Could you check a few things on this model? Use its own coordinates, in mm. A direction names the side the tool comes from. Give positions to 0.01 mm unless a question says otherwise; leave off trailing zeros. Order: outer loops, then holes, each group sorted by start corner. A loop starts at its lowest first (then second) coordinate and runs counter-clockwise, first axis right, second up.
(1) Imagine slicing it at A-A, the plane z = 10. Write out the boundary of the cut face in (x, y).
(2) Imagine slicing it at C-C, the plane z = 67.5. Write out the boundary of the cut face in (x, y).
(3) Imagine slicing it at D-D, the plane y = 195. Write out the boundary of the cut face in (x, z), then the cut area to 3 significant figures.
(4) If we mould it in two halves opening along Z, with no side actions, what happens to faces 1 (the cylindrical face through (-175.427, 194.12, 88.496)), 2 (the cylindrical face through (-215.896, 224.268, 60.035)), 3 (the flat face through (-177.399, 209, 45))? For each: released by +Z, released by -Z, zero draft, split by the parting line, or undercut.
(5) If I drill on probe 1 along Z at (x, y) = (-183, 211); probe 2 along Y at (x, z) = (-174.7, 80); probe 3 along X at (y, z) = (222.5, 67), over which ranges is the centre line in solid material (lowest first)?
(6) Will these pins go through, and if not, where does the flat tip stop? pin 1 (4 mm diameter, centred on x = -190.45, y = 215.17, fed in from +Z); pin 2 (1.4 mm diameter, centred on x = -202.62, y = 206.36, fed in from +Z); pin 3 (3 mm diameter, centred on x = -196.676, y = 214.585, fed in from -Z).
(7) Imagine slicing it at B-B, the plane y = 204. Write out the boundary of the cut face in (x, z), then the cut area to 3 significant figures.
(8) On a 3-axis mill with a long thin cutter (end or side, diameter ignored), from which of +Z, -Z, +X, -X, +Y, -Y can I reach the whole of each face in a straight line? I mean faces 4 (the flat face through (-175, 209, 0)), 5 (the cylindrical face through (-189.717, 216.122, 59.965)), 6 (the flat face through (-197, 209, 32.5)), 7 (the flat face through (-175, 209, 90)), 8 (the flat face through (-177.399, 209, 76)). Say none if no direction works.
Autodesk Inventor part; units mm, degrees
ref_plane "YZ Plane" through (0, 0, 0) normal (1, 0, 0) x (0, 1, 0)
ref_plane "XZ Plane" through (0, 0, 0) normal (0, 1, 0) x (-1, 0, 0)
ref_plane "XY Plane" through (0, 0, 0) normal (0, 0, 1) x (1, 0, 0)
sketch "Szkic1" plane through (0, 0, 0) normal (0, 0, 1) x (1, 0, 0)
  circle A0 centre (0, 0) radius 55 construction
  circle A1 centre (137.9996, 0.347) radius 55 construction
  circle A2 centre (275.9991, 0.6941) radius 55 construction
  line L0 (-173.3991, 195.8773) -> (-173.4121, 201.0636) construction
  line L1 (-173.3991, 247) -> (-173.3991, -116) construction
  line L2 (275.9991, -54.3059) -> (-673, -54.3059) construction
  line L3 (-488.3991, -4.3059) -> (-438.3991, -4.3059) construction
  line L4 (-438.3991, -4.3059) -> (-438.3991, -54.3059) construction
  line L5 (-438.3991, -54.3059) -> (-488.3991, -54.3059) construction
  line L6 (-488.3991, -54.3059) -> (-488.3991, -4.3059) construction
  line L7 (-438.4326, 222.6941) -> (233, 222.6941) construction
  line L8 (-438.4326, 192.6941) -> (378, 192.6941) construction
  line L9 (-476, 207.6941) -> (256, 207.6941) construction
  line L10 (-173.3991, 192.6941) -> (-177.3991, 192.6941)
  line L11 (-177.3991, 192.6941) -> (-177.3991, 225.6941)
  line L12 (-177.3991, 225.6941) -> (-173.3991, 225.6941)
  line L13 (-173.3991, 225.6941) -> (-173.3991, 192.6941)
  point P0 (15, -3)
  dimension "d0" = 50
  dimension "d1" = 50
  dimension "d2" = 265
  dimension "d3" = 277
  dimension "d4" = 30
  dimension "d5" = 15
  dimension "d6" = 4
  dimension "d62" = 33
extrude "Wyciągnięcie proste1" add sketch "Szkic1" along normal blind 90
sketch "Szkic2" plane through (-177.3991, 192.6941, 0) normal (-1, 0, 0) x (0, 0, 1)
  line L0 (90, 0) -> (90, 33)
  line L1 (0, 0) -> (0, 33)
  line L2 (0, 0) -> (0, 33)
  line L3 (0, 0) -> (90, 0)
  line L4 (90, 33) -> (90, 0)
  line L5 (0, 33) -> (90, 33)
  line L6 (0, 33) -> (90, 33)
  line L7 (0, 0) -> (90, 0)
  line L8 (57.5, 33) -> (62.5, 33)
  line L9 (62.5, 33) -> (62.5, 0)
  line L10 (62.5, 0) -> (57.5, 0)
  line L11 (57.5, 0) -> (57.5, 33)
  line L12 (32.5, 33) -> (27.5, 33)
  line L13 (27.5, 33) -> (27.5, 0)
  line L14 (27.5, 0) -> (32.5, 0)
  line L15 (32.5, 0) -> (32.5, 33)
  point P0 (0, -192.6941)
  point P1 (80, 16)
  point P2 (10, 16)
  dimension "d9" = 10
  dimension "d10" = 10
  dimension "d11" = 5
  dimension "d12" = 5
  dimension "d13" = 17.5
  dimension "d14" = 17.5
extrude "Wyciągnięcie proste2" add sketch "Szkic2" along normal blind 40 contours L3 L11 L5 L9 | L3 L13 L5 L15
fillet "Zaokrąglenie1" radius 5 8 edges at (-217.3991, 192.6941, 60) (-217.3991, 225.6941, 60) (-217.3991, 225.6941, 30) (-217.3991, 192.6941, 30) (-175.3991, 192.6941, 90) (-175.3991, 225.6941, 90) (-175.3991, 225.6941, 0) (-175.3991, 192.6941, 0)
sketch "Szkic3" plane through (-177.3991, 192.6941, 62.5) normal (0, 0, 1) x (1, 0, 0)
  line L0 (-298.6009, 15) -> (433.3991, 15) construction
  line L1 (-40, 5) -> (-40, 28)
  line L2 (-311, -197) -> (-261, -197) construction
  line L3 (-261, -247) -> (-311, -247) construction
  line L4 (-497, -197) -> (104, -197) construction
  line L5 (-221, 86) -> (-221, -341.1695) construction
  line L6 (-246, 90.4419) -> (-246, -336.7276) construction
  line L7 (-296, 88) -> (-296, -339.1695) construction
  line L8 (-271, 89) -> (-271, -338.1695) construction
  line L9 (4, 54.3059) -> (4, -308.6941) construction
  line L10 (-221, -197) -> (144.5683, 199.6805) construction
  line L11 (-246, -197) -> (156.8943, 188.8706) construction
  line L12 (-271, -197) -> (64.3345, 90.4296) construction
  line L13 (-296, -197) -> (182.0787, 173.8291) construction
  line L14 (-196, -338.1695) -> (-196, 81) construction
  line L15 (-171, -340.9749) -> (-171, 78.1946) construction
  line L16 (-296, -333) -> (-296, 85.2632) construction
  line L17 (-321, 80.9017) -> (-321, -346.2678) construction
  line L18 (-196, -197) -> (27.7781, 83.0658) construction
  circle A0 centre (-33, 7) radius 26.5 construction
  circle A1 centre (-33, 7) radius 24 construction
  circle A2 centre (-33, 7) radius 19 construction
  circle A3 centre (-33, 7) radius 25.25 construction
  circle A4 centre (-33, 7) radius 21.5 construction
  circle A5 centre (-33, 7) radius 20.25 construction
  circle A6 centre (-33, 7) radius 31.5 construction
  circle A7 centre (-33, 7) radius 16.5 construction
  circle A8 centre (-33, 7) radius 15.25 construction
  circle A9 centre (-33, 7) radius 14 construction
  circle A10 centre (-33, 7) radius 11.5 construction
  circle A11 centre (-33, 7) radius 10.25 construction
  circle A12 centre (-33, 7) radius 9 construction
  point P0 (177.3991, -192.6941)
  point P1 (-33, 15)
  point P2 (-13.0484, 22.4757)
  point P3 (-21.9865, 17.5482)
  point P4 (-25.2176, 13.6706)
  point P5 (-19.277, 21.891)
  point P6 (-17.2382, 26.7264)
  dimension "d33" = 40.5
  dimension "d36" = 30.5
  dimension "d46" = 20.5
  dimension "d18" = 7
  dimension "d19" = 8
  dimension "d20" = 225
  dimension "d21" = 250
  dimension "d22" = 275
  dimension "d24" = 200
  dimension "d25" = 175
  dimension "d26" = 300
  dimension "d27" = 325
  dimension "d28" = 53
  dimension "d29" = 48
  dimension "d30" = 38
  dimension "d31" = 50.5
  dimension "d32" = 43
  dimension "d34" = 63
  dimension "d35" = 33
  dimension "d37" = 28
  dimension "d45" = 23
  dimension "d47" = 18
hole "Otwór2" at (-190.4475, 215.1698, 62.5) at (-199.3855, 210.2423, 62.5) at (-202.6167, 206.3647, 62.5) at (-196.676, 214.585, 62.5) at (-194.6373, 219.4204, 62.5) direction (0, 0, -1) diameter 2.4 depth 8 tip angle 118
hole "Otwór3" at (-210.3991, 199.6941, 62.5) direction (0, 0, -1) diameter 3.9 end through all
sketch "Szkic4" plane through (-173.3991, 197.6941, 0) normal (1, 0, 0) x (0, 0, -1)
  line L0 (-90, 23) -> (-90, 0)
  line L1 (-5, 28) -> (-85, 28)
  point P0 (0, -197.6941)
  point P1 (-80, 11.5)
  point P2 (-10, 11.5)
  dimension "d63" = 70
  dimension "d64" = 10
  dimension "d65" = 16.5
hole "Otwór4" at (-173.3991, 209.1941, 80) at (-173.3991, 209.1941, 10) direction (-1, 0, 0) diameter 4.5 depth 8 tip angle 118
equation "\"d5\" = 0.5 * d4"
properties part number "Czesc_do_Ramy"
Answer block:
1. outline: (-177.4, 192.69) - (-173.4, 192.69) - (-173.4, 206.94) - (-177.4, 206.94) - close; (-177.4, 211.44) - (-173.4, 211.44) - (-173.4, 225.69) - (-177.4, 225.69) - close
2. outline: (-177.4, 192.69) - (-173.4, 192.69) - (-173.4, 225.69) - (-177.4, 225.69) - close
3. outline: (-216.61, 27.5) - (-177.4, 27.5) - (-177.4, 0.79) - (-173.4, 0.79) - (-173.4, 89.21) - (-177.4, 89.21) - (-177.4, 62.5) - (-216.61, 62.5) - (-216.61, 57.5) - (-177.4, 57.5) - (-177.4, 32.5) - (-216.61, 32.5) - close
3. area: 746 mm2
4. face 1: released by +Z
4. face 2: zero draft
4. face 3: undercut
5. probe 1: z = 27.5 to 32.5, 57.5 to 62.5
5. probe 2: y = 192.69 to 206.94, 211.44 to 225.69
5. probe 3: x = -177.4 to -173.4
6. pin 1: stops at z = 62.5
6. pin 2: stops at z = 32.5
6. pin 3: stops at z = 27.5
7. outline: (-217.4, 27.5) - (-177.4, 27.5) - (-177.4, 0) - (-173.4, 0) - (-173.4, 90) - (-177.4, 90) - (-177.4, 62.5) - (-217.4, 62.5) - (-217.4, 57.5) - (-177.4, 57.5) - (-177.4, 32.5) - (-217.4, 32.5) - close
7. area: 760 mm2
8. face 4: -Z, +X, -X, +Y, -Y
8. face 5: +Z
8. face 6: -X, +Y, -Y
8. face 7: +Z, +X, -X, +Y, -Y
8. face 8: +Z, -X, +Y, -Y
